from build123d import *

# Parameters (mm, degrees)
SKETCH1_R                   = 28.575
OD_DON_T_CARE_DEPTH         = 57.15
SKETCH3_W                   = 25.4
SKETCH3_H                   = 44.577
SLOT_DEPTH                  = 50.8
SKETCH4_R                   = 7.9375
F_5_8_THROUGH_HOLE_DEPTH    = 61.167850045
SKETCH5_OUTSIDE_W           = 78.948
SKETCH5_OUTSIDE_H           = 78.948
SKETCH5_OUTSIDE_W_2         = 53.975
SKETCH5_OUTSIDE_H_2         = 51.195336702
FLAT_SURFACE_DEPTH          = 25.4
SKETCH2_R                   = 3.175
F_1_4_THROUGH_HOLE_DEPTH    = 38.1
SKETCH7_R                   = 1.984375
F_10_32_THREADED_HOLE_DEPTH = 77.067593297


with BuildPart() as part:
    # Sketch1 → OD Don't Care (new body)
    with BuildSketch(Plane.XY):
        Circle(SKETCH1_R)
    extrude(amount=OD_DON_T_CARE_DEPTH)

    # Sketch3 → Slot (cut, symmetric)
    with BuildSketch(Plane(origin=(0, 0, 0), x_dir=(1, 0, 0), z_dir=(0, 1, 0))):
        with Locations((0, -34.8615)):
            Rectangle(SKETCH3_W, SKETCH3_H)
    extrude(amount=SLOT_DEPTH, both=True, mode=Mode.SUBTRACT)

    # Sketch4 → 5/8" Through Hole (cut, through all)
    with BuildSketch(Plane.XY.offset(12.573)):
        Circle(SKETCH4_R)
    extrude(amount=-F_5_8_THROUGH_HOLE_DEPTH, mode=Mode.SUBTRACT)

    # Sketch5 outside → Flat Surface (cut)
    with BuildSketch(Plane.XY.offset(57.15)):
        Rectangle(SKETCH5_OUTSIDE_W, SKETCH5_OUTSIDE_H)
        with Locations((-1.5875, 0)):
            Rectangle(SKETCH5_OUTSIDE_W_2, SKETCH5_OUTSIDE_H_2, mode=Mode.SUBTRACT)
    extrude(amount=-FLAT_SURFACE_DEPTH, mode=Mode.SUBTRACT)

    # Sketch2 → 1/4" Through Hole (cut)
    with BuildSketch(Plane(origin=(25.4, 0, 0), x_dir=(0, 0, -1), z_dir=(1, 0, 0))):
        with Locations((-44.45, 0)):
            Circle(SKETCH2_R)
    extrude(amount=-F_1_4_THROUGH_HOLE_DEPTH, mode=Mode.SUBTRACT)

    # Sketch7 → 10-32 Threaded Hole (cut, through all)
    with BuildSketch(Plane(origin=(-12.7, 0, 0), x_dir=(0, 0, -1), z_dir=(1, 0, 0))):
        with Locations((-44.45, 0)):
            Circle(SKETCH7_R)
    extrude(amount=-F_10_32_THREADED_HOLE_DEPTH, mode=Mode.SUBTRACT)


solid = part.part
Source: CAD feature listing. Evaluate the final solid. Frame: model axes, mm. A direction names the side the tool comes from. Give positions to 0.01 mm unless a question says otherwise; leave off trailing zeros. Write each loop counter-clockwise with the first axis right and the second up, starting at its lowest first coordinate (ties: lowest second). Pieces come first, ordered by that corner, then holes. Notation, with made-up numbers: (-17, 73) -> (24, 73) arc R18 cw to (24, 96) -> close; hole circle Ø1 at (51.5, 9). An arc over 180 degrees is marked (long way). Return JSON: item names as keys, results as strings. Group by question number.
1. Pin query (flat end, axial travel): pin 1 Ø2.5 at (x, y) = (27.5, -2) entering from +Z; pin 2 Ø6 at (x, y) = (-22, 20.5) entering from +Z; pin 3 Ø4.5 at (y, z) = (0, 44.45) entering from +X; pin 4 Ø5 at (y, z) = (-9.5, 35) entering from -X. Return the tip coordinate at first contact, or that it passes through.
2. Material intervals for line 1 (Y direction, x = 0, z = 3) (1 decimal); line 2 (Y direction, x = 21, z = 43.5); line 3 (Z direction, x = -6.5, y = 13.5), sorted ascending. Write a range as from..to.
3. Section B-B, the plane y = 0. Count the separate pieces of the cut face and the enclosed holes in it, then the cut area to 3 significant figures.
4. Section C-C, the plane z = 44.45. Output: boundary loops of the cut face in (x, y) (3 decimals), then the cut area to 3 significant figures.
5. Access query for faces 4 (the face through (8.3, 0.4, 12.573)), 5 (the face through (27, 0, 31.75)), 6 (the face through (-19, 0, 57.15)). Directions: +Z, -Z, +X, -X, +Y, -Y. A direction counts if a zero-diameter tool reaches every point of the face in a straight line with its end or side. Return the directions, or none.
6. Mould query, pull axis Y, two halves, no side actions, for faces 1 (the face through (25.4, -3, 47)), 2 (the face through (-28.547, 1.256, 21.825)), 3 (the face through (19.14, 0.95, 41.42)). Classes: +Y half, -Y half, draft (parallel to the pull), parting line (faces both ways), or undercut.
7. Section D-D, the plane y = -6. Output: boundary loops of the cut face in (x, z).
8. Section A-A, the plane x = 0. Output: boundary loops of the cut face in (y, z) (1 decimal), then the cut area to 3 significant figures.
Determined:
{
 "1": {"pin 1": "stops at z = 31.75", "pin 2": "stops at z = 57.15", "pin 3": "stops at x = -12.7", "pin 4": "stops at x = -27.7"},
 "2": {"line 1": "y = -28.6..-7.9, 7.9..28.6", "line 2": "y = -19.38..-3.03, 3.03..19.38", "line 3": "z = 0..12.57"},
 "3": {"separate pieces": "4", "enclosed holes": "0", "area": "1,710 mm2"},
 "4": {"outline": "(-28.506, -1.984) arc R28.575 ccw to (-12.7, -25.598) -> (-12.7, -1.984) -> close; (-28.506, 1.984) -> (-12.7, 1.984) -> (-12.7, 25.598) arc R28.575 ccw to start; (12.7, -25.598) arc R28.575 ccw to (25.4, -13.091) -> (25.4, -3.175) -> (12.7, -3.175) -> close; (12.7, 3.175) -> (25.4, 3.175) -> (25.4, 13.091) arc R28.575 ccw to (12.7, 25.598) -> close", "area": "963 mm2"},
 "5": {"face 4": "+Z, +Y, -Y", "face 5": "+Z, +X, +Y, -Y", "face 6": "+Z, +X, -X, +Y, -Y"},
 "6": {"face 1": "draft", "face 2": "parting line", "face 3": "undercut"},
 "7": {"outline": "(-27.94, 0) -> (-5.2, 0) -> (-5.2, 12.57) -> (-12.7, 12.57) -> (-12.7, 57.15) -> (-27.94, 57.15) -> close; (5.2, 0) -> (27.94, 0) -> (27.94, 31.75) -> (25.4, 31.75) -> (25.4, 57.15) -> (12.7, 57.15) -> (12.7, 12.57) -> (5.2, 12.57) -> close"},
 "8": {"outline": "(-28.6, 0) -> (-7.9, 0) -> (-7.9, 12.6) -> (-28.6, 12.6) -> close; (7.9, 0) -> (28.6, 0) -> (28.6, 12.6) -> (7.9, 12.6) -> close", "area": "519 mm2"}
}
